Check sheet for the modelled part. Datum: model origin and axes. Units: mm. Face numbers are marked on the shaded views. A direction names the side the tool comes from. Give positions to 0.01 mm unless a question says otherwise; leave off trailing zeros. Loops run counter-clockwise (first coordinate to the right, second up) from the corner with the lowest first, then second, coordinate; pieces in that order, holes last. Notation, with made-up numbers: M 25,-3 L 76,-3 A24 ccw 76,30 Z; hole C 86.25,-18.75 d10. An arc over 180 degrees is marked long. Use one line per item in the form item = value.
from build123d import *

# Parameters (mm, degrees)
F0_R      = 40
F1_DEPTH  = 160
F3_R      = 10
F1_FACE_R = 40
F5_DEPTH  = 40
F6_W      = 80
F6_H      = 20
F7_DEPTH  = 40
F8_R      = 18
F9_DEPTH  = 20
F10_R     = 20
F10_R_2   = 18
F11_DEPTH = 50


with BuildPart() as f1:
    # F0 (on Top) → F1 (new body)
    with BuildSketch(Plane.XY):
        Circle(F0_R)
    extrude(amount=-F1_DEPTH)

    # F3 (on offset) → F4 section 0
    with BuildSketch(Plane(origin=(0, 0, -320), x_dir=(1, 0, 0), z_dir=(0, 0, -1))):
        Circle(F3_R)
    # F1_face (on face) → F4 section 1
    with BuildSketch(Plane(origin=(0, 0, -160), x_dir=(1, 0, 0), z_dir=(0, 0, -1))):
        Circle(F1_FACE_R)
    loft()

    # F5 (add): a face of the model
    f5_faces = [f1.faces().sort_by_distance(p)[0] for p in [
        (0, 0, -320),
    ]]
    extrude(f5_faces, amount=F5_DEPTH)

    # F6 (on Top) → F7 (join)
    with BuildSketch(Plane.XY):
        with Locations((-40, 30)):
            Rectangle(F6_W, F6_H)
    extrude(amount=-F7_DEPTH)

    # F8 (on face) → F9 (join)
    with BuildSketch(Plane.XY):
        Circle(F8_R)
    extrude(amount=F9_DEPTH)

    # F10 (on face) → F11 (cut)
    with BuildSketch(Plane.XY):
        Circle(F10_R)
        Circle(F10_R_2, mode=Mode.SUBTRACT)
    extrude(amount=-F11_DEPTH, mode=Mode.SUBTRACT)


solid = f1.part
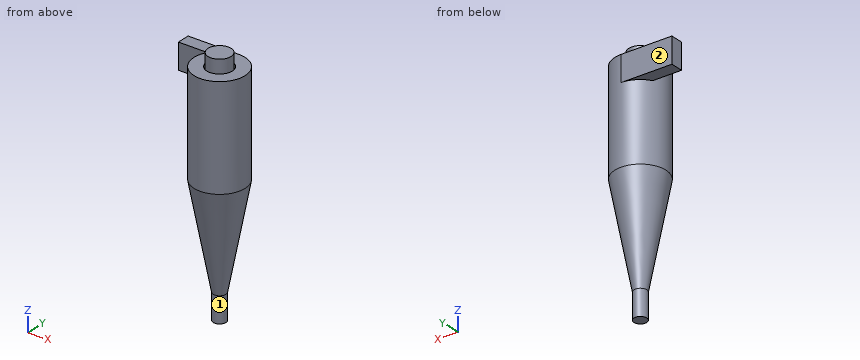
1) Scan lines: line 1 (Y direction, x = 0, z = -27); line 2 (X direction, y = -9, z = -6.5); line 3 (Y direction, x = -63.5, z = -15). Record each from-to range of solid material in increasing order.
Evaluation:
line_1 = -40 to -20, -18 to 18, 20 to 40
line_2 = -38.97 to -17.86, -15.59 to 15.59, 17.86 to 38.97
line_3 = 20 to 40
2) Depth check by flat-ended pin: pin 1 Ø1.5 at (y, z) = (-26.5, -103.5) entering from -X; pin 2 Ø1 at (x, y) = (-32.5, 23.5) entering from +Z; pin 3 Ø20 at (x, z) = (-63, -18.5) entering from -Y. Enter the tip coordinate at first touch or a pass-through.
Evaluation:
pin_1 = -30.61
pin_2 = 0
pin_3 = 20
3) Section check A-A (z = -4.5). Record the cut outline in (x, y).
Evaluation:
outline = M -80,20 L -34.64,20 A40 ccw long 0,40 L -80,40 Z; C 0,0 d36; hole C 0,0 d40
4) Section check C-C (z = -152.5). Record the cut outline in (x, y).
Evaluation:
outline = C 0,0 d80
5) Set-up check for the marked faces 1 and 2: record each of +Z, -Z, +X, -X, +Y, -Y from which the full face is reachable in a straight line by a thin tool's end or side.
Evaluation:
face_1 = -Z
face_2 = +Z, -Z, +X, -X, +Y
6) Section check B-B (x = -69). Record the cut outline in (y, z).
Evaluation:
outline = M 20,-40 L 40,-40 L 40,0 L 20,0 Z
